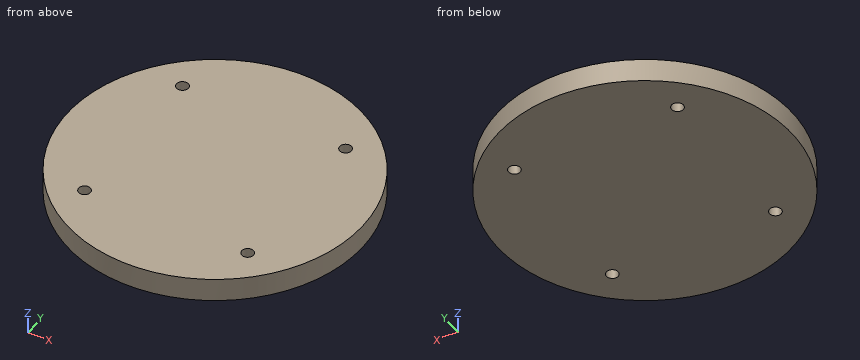
Autodesk Inventor part; units mm, degrees
ref_plane "YZ Plane" through (0, 0, 0) normal (1, 0, 0) x (0, 1, 0)
ref_plane "XZ Plane" through (0, 0, 0) normal (0, 1, 0) x (-1, 0, 0)
ref_plane "XY Plane" through (0, 0, 0) normal (0, 0, 1) x (1, 0, 0)
ref_plane "Work Plane1" through (0, 0, 0) normal (0, 0, 1) x (1, 0, 0)
sketch "Sketch1" plane through (0, 0, 0) normal (0, 0, 1) x (1, 0, 0)
  circle A0 centre (-20.75, 20.75) radius 1.5
  circle A1 centre (-20.75, -20.75) radius 1.5
  circle A2 centre (20.75, 20.75) radius 1.5
  circle A3 centre (20.75, -20.75) radius 1.5
  circle A4 centre (0, 0) radius 37.5402
extrude "Plate1" add sketch "Sketch1" along normal blind 6
equation "\"d0\" = Thickness"
equation "\"BendRadius\" = Thickness"
equation "\"BendReliefWidth\" = Thickness"
equation "\"BendReliefDepth\" = 0.5 * Thickness"
equation "\"CornerReliefSize\" = 4 * Thickness"
equation "\"MinimumRemnant\" = 2 * Thickness"
equation "\"TransitionRadius\" = BendRadius"
equation "\"JacobiRadiusSize\" = BendRadius"
equation "\"GapSize\" = Thickness"
properties part number "spacer lidar" material "Wood (Birch)"
The model under review builds one solid part; all positions refer to its coordinate system, in mm. Give positions to 0.01 mm unless a question says otherwise; leave off trailing zeros. Write each loop counter-clockwise with the first axis right and the second up, starting at its lowest first coordinate (ties: lowest second). Pieces come first, ordered by that corner, then holes. Notation, with made-up numbers: (-32, 66.25) - (-15, 66.25) arc R15 ccw to (-15, 88.25) - close; hole circle Ø7 at (-20.5, -23). An arc over 180 degrees is marked (long way). Answer in a Markdown table with one row per item. Add a question column.
1. Wall thickness on line 1 along Y through (x, z) = (-20.75, 3); line 2 along Y through (x, z) = (20.5, 2); line 3 along Y through (x, z) = (-1, 1.25): over which ranges is each line inside the solid? List them lowest first. Write a range as [from, to].
2. We need section B-B on z = 1.85. Write out the cut boundary in (x, y), then the cut area to 3 significant figures.
3. We need section D-D on x = 9. Write out the cut boundary in (y, z), then the cut area to 3 significant figures.
4. Insertion check: P1, Ø3, axis at x = -19, z = 1, coming from the +Y side; P2, Ø4, axis at x = -20.75, y = -20.75, coming from the -Z side; P3, Ø3, axis at y = 17.5, z = 3.5, coming from the +X side; P4, Ø1, axis at x = 21.5, z = 5.5, coming from the -Y side. Each pin has a flat end and moves straight along its axis. Give the tip position at first contact, or say it passes through.
5. We need section A-A on x = 20.75. Write out the cut boundary in (y, z).
Ans:
| question | item | result |
|---|---|---|
| 1 | line 1 | y = [-31.28, -22.25], [-19.25, 19.25], [22.25, 31.28] |
| 1 | line 2 | y = [-31.45, -22.23], [-19.27, 19.27], [22.23, 31.45] |
| 1 | line 3 | y = [-37.53, 37.53] |
| 2 | outline | circle Ø75.08 at (0, 0); hole circle Ø3 at (-20.75, -20.75); hole circle Ø3 at (-20.75, 20.75); hole circle Ø3 at (20.75, -20.75); hole circle Ø3 at (20.75, 20.75) |
| 2 | area | 4,400 mm^2 |
| 3 | outline | (-36.45, 0) - (36.45, 0) - (36.45, 6) - (-36.45, 6) - close |
| 3 | area | 437 mm^2 |
| 4 | P1 | stops at y = 33.21 |
| 4 | P2 | stops at z = 0 |
| 4 | P3 | stops at x = 33.96 |
| 4 | P4 | stops at y = -31.12 |
| 5 | outline | (-31.28, 0) - (-22.25, 0) - (-22.25, 6) - (-31.28, 6) - close; (-19.25, 0) - (19.25, 0) - (19.25, 6) - (-19.25, 6) - close; (22.25, 0) - (31.28, 0) - (31.28, 6) - (22.25, 6) - close |
